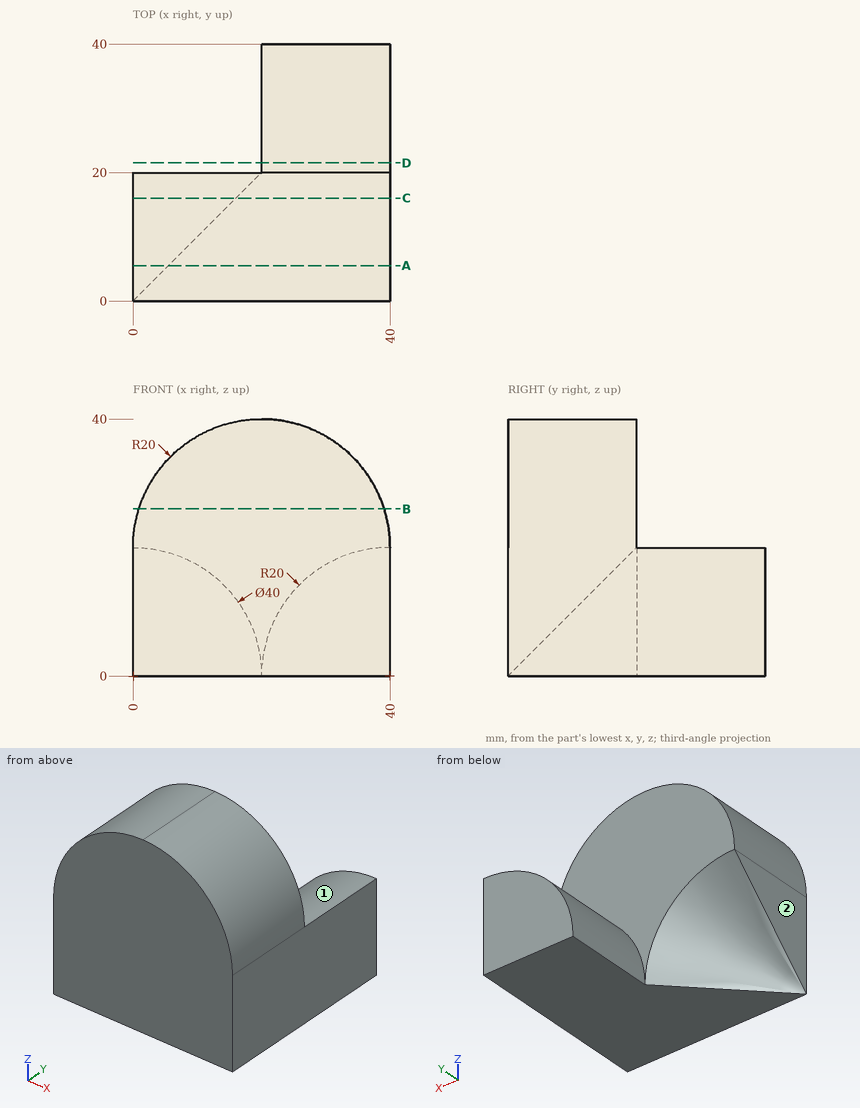
Answer from the drawing. Dimensions are ordinates in mm from the lowest x, y and z of the part. A direction names the side the tool comes from. Coordinates: 2 decimals unless noted, no trailing zeros. Write each loop counter-clockwise with the first axis right and the second up, starting at its lowest first coordinate (ties: lowest second). Pieces come first, ordered by that corner, then holes. Notation, with made-up numbers: (19, 24) - (76, 24) arc R25 cw to (76, 56) - close; hole circle Ø4 at (-22.5, 21). An arc over 180 degrees is marked (long way). Return JSON: item names as keys, results as strings. Group by question number.
Q1. The part is cut by section A-A on y = 5.5. Write down the section's boundary in (x, z).
Q2. The part is cut by section D-D on y = 21.5. Write down the section's boundary in (x, z).
Q3. The part is cut by section C-C on y = 16. Write down the section's boundary in (x, z), and give its area (3 significant figures).
Q4. Which of the six approach directions +Z, -Z, +X, -X, +Y, -Y give full straight-line access (tool end or side, diameter ignored) to the marked faces 1 and 2?
Q5. Flat-ended cylindrical pins translate along their axes: pin 1 Ø6 at (y, z) = (31.5, 10.5) entering from -X; pin 2 Ø6 at (x, y) = (4.5, 17) entering from -Z; pin 3 Ø3 at (x, y) = (26, 12) entering from +Z; pin 4 Ø12 at (x, y) = (6.5, 31) entering from +Z. Find the tip coordinate at first contact, or state that the pin passes through.
Q6. The part is cut by section B-B on z = 26. Write down the section's boundary in (x, y).
Q7. Find the intervals of material crossed by line 1 along Y through (x, z) = (3.5, 31); line 2 along Z through (x, y) = (23, 19); line 3 along Z through (x, y) = (38.5, 35.5), in increasing order. Write a range as [from, to].
Evaluation:
{
 "1": {"outline": "(0, 5.5) arc R5.5 cw to (5.5, 0) - (40, 0) - (40, 20) arc R20 ccw to (0, 20) - close"},
 "2": {"outline": "(20, 0) - (40, 0) - (40, 20) arc R20 ccw to start"},
 "3": {"outline": "(0, 16) arc R16 cw to (16, 0) - (40, 0) - (40, 20) arc R20 ccw to (0, 20) - close", "area": "1,230 mm2"},
 "4": {"face 1": "+Z, -X, +Y", "face 2": "+Z, -Z, -X, +Y, -Y"},
 "5": {"pin 1": "stops at x = 21.46", "pin 2": "stops at z = 13.06", "pin 3": "stops at z = 39.49", "pin 4": "passes through"},
 "6": {"outline": "(0.92, 0) - (39.08, 0) - (39.08, 20) - (0.92, 20) - close"},
 "7": {"line 1": "y = [0, 20]", "line 2": "z = [0, 39.77]", "line 3": "z = [0, 19.94]"}
}
